from build123d import *

# Parameters (mm, degrees)
RESSALTO_EXTRUS_O1_DEPTH   = 10
ESBO_O3_W                  = 8
ESBO_O3_H                  = 6
CORTE_EXTRUS_O2_DEPTH      = 1
CORTE_EXTRUS_O2_DEPTH_BACK = 57.536791537
CORTE_EXTRUS_O1_REACH      = 63.225
ESBO_O2_R                  = 1.7
ESBO_O6_W                  = 10
ESBO_O6_H                  = 10
ESBO_O6_R                  = 1.7
RESSALTO_EXTRUS_O2_DEPTH   = 5
CORTE_EXTRUS_O5_DEPTH      = 4


with BuildPart() as part:
    # Esboço1 → Ressalto-extrusão1 (new body)
    with BuildSketch(Plane.XY):
        Polygon((0, 0), (0, -26), (6, -26), (6, -6), (26, -6), (26, -26), (32, -26), (32, 35.240055442), (56.536791537, 70.282225368), (51.621879272, 73.723683986), align=None)
        Polygon((26, 0), (26, 26.671167402), (7.324647533, 0), align=None, mode=Mode.SUBTRACT)
    extrude(amount=RESSALTO_EXTRUS_O1_DEPTH)

    # Esboço3 → Corte-extrusão2 (cut, two sides)
    with BuildSketch(Plane.ZY) as corte_extrus_o2_sk:
        with Locations((4, -16)):
            Rectangle(ESBO_O3_W, ESBO_O3_H)
    extrude(amount=CORTE_EXTRUS_O2_DEPTH, mode=Mode.SUBTRACT)
    extrude(corte_extrus_o2_sk.sketch, amount=-CORTE_EXTRUS_O2_DEPTH_BACK, mode=Mode.SUBTRACT)

    # Esboço2 → Corte-extrusão1 (cut, up to next)
    with BuildSketch(Plane(origin=(0, 0, 0), x_dir=(0, 0, 1), z_dir=(-0.819152044, 0.573576436, 0)), mode=Mode.PRIVATE) as corte_extrus_o1_sk1:
        with Locations((5, 85)):
            Circle(ESBO_O2_R)
    corte_extrus_o1_tool1 = extrude(corte_extrus_o1_sk1.sketch, amount=-CORTE_EXTRUS_O1_REACH, mode=Mode.PRIVATE) & part.part
    add(corte_extrus_o1_tool1.solids().sort_by_distance((48.753997, 69.627924, 5))[0], mode=Mode.SUBTRACT)
    # Esboço2 → Corte-extrusão1 (cut, up to next)
    with BuildSketch(Plane(origin=(0, 0, 0), x_dir=(0, 0, 1), z_dir=(-0.819152044, 0.573576436, 0)), mode=Mode.PRIVATE) as corte_extrus_o1_sk2:
        with Locations((5, 20)):
            Circle(ESBO_O2_R)
    corte_extrus_o1_tool2 = extrude(corte_extrus_o1_sk2.sketch, amount=-CORTE_EXTRUS_O1_REACH, mode=Mode.PRIVATE) & part.part
    add(corte_extrus_o1_tool2.solids().sort_by_distance((11.471529, 16.383041, 5))[0], mode=Mode.SUBTRACT)

    # Esboço6 → Ressalto-extrusão2 (add)
    with BuildSketch(Plane(origin=(0, 0, 0), x_dir=(0, 0, 1), z_dir=(-0.819152044, 0.573576436, 0))):
        with Locations((5, 85)):
            Rectangle(ESBO_O6_W, ESBO_O6_H)
        with Locations((5, 85)):
            Circle(ESBO_O6_R, mode=Mode.SUBTRACT)
        with Locations((5, 20)):
            Rectangle(ESBO_O6_W, ESBO_O6_H)
        with Locations((5, 20)):
            Circle(ESBO_O6_R, mode=Mode.SUBTRACT)
    extrude(amount=RESSALTO_EXTRUS_O2_DEPTH)

    # Esboço7 → Corte-extrusão5 (cut)
    with BuildSketch(Plane(origin=(4.914912266, -3.441458618, 0), x_dir=(0, 0, -1), z_dir=(0.819152044, -0.573576436, 0))):
        Polygon((-2.15, 83.354551733), (-2.15, 86.645448267), (-5, 88.290896534), (-7.85, 86.645448267), (-7.85, 83.354551733), (-5, 81.709103466), align=None)
        Polygon((-2.15, 18.354551733), (-2.15, 21.645448267), (-5, 23.290896534), (-7.85, 21.645448267), (-7.85, 18.354551733), (-5, 16.709103466), align=None)
    extrude(amount=-CORTE_EXTRUS_O5_DEPTH, mode=Mode.SUBTRACT)


solid = part.part
Design review of the part built by this model. Coordinates are the model's own, in mm. A direction names the side the tool comes from. Give positions to 0.01 mm unless a question says otherwise; leave off trailing zeros. Loops run counter-clockwise (first coordinate to the right, second up) from the corner with the lowest first, then second, coordinate; pieces in that order, holes last. Notation, with made-up numbers: (-16.5, -10.75) - (28.5, -10.75) arc R8 ccw to (28.5, -6.75) - close; hole circle Ø4 at (63, 53). An arc over 180 degrees is marked (long way). Write item = value, one per line.
1) Take a section at A-A on y = -8. State the section outline as (x, z) points.
Result sheet:
outline = (0, 0) - (6, 0) - (6, 10) - (0, 10) - close; (26, 0) - (32, 0) - (32, 10) - (26, 10) - close
2) Take a section at B-B on x = 20. State the section outline as (y, z) points, and give its area (3 significant figures).
Result sheet:
outline = (-6, 0) - (0, 0) - (0, 10) - (-6, 10) - close; (18.1, 0) - (28.56, 0) - (28.56, 10) - (18.1, 10) - close
area = 165 mm2
3) Take a section at C-C on x = 29. State the section outline as (y, z) points, and give its area (3 significant figures).
Result sheet:
outline = (-26, 0) - (-19, 0) - (-19, 8) - (-13, 8) - (-13, 0) - (41.42, 0) - (41.42, 10) - (-26, 10) - close
area = 626 mm2
4) Take a section at D-D on y = 59. State the section outline as (x, z) points, and give its area (3 significant figures).
Result sheet:
outline = (41.31, 0) - (48.64, 0) - (48.64, 10) - (41.31, 10) - close
area = 73.2 mm2
5) To check wall thickness, follow line 1 (Y direction, x = 14.5, z = 2.25); line 2 (X direction, y = -14, z = 8.25); line 3 (Z direction, x = 12, y = 17). State the ranges of each line that lie inside material, in increasing order.
Result sheet:
line_1 = -6 to 0, 10.25 to 12.18, 16.34 to 20.71
line_2 = 0 to 6, 26 to 32
line_3 = 0 to 3.5, 6.5 to 10
6) Draft analysis for pull direction X (two halves, no side actions). For faces 1 (the face through (3, -22, 0)), 2 (the face through (13, 12, 6)), 3 (the face through (0, -12.8, 4.9)), state which applies: +X half, -X half, draft (parallel to the pull), parting line (faces both ways), or undercut.
Result sheet:
face_1 = draft
face_2 = undercut
face_3 = -X half
7) Clearance check with flat-ended pins moving along their axes: pin 1 Ø2 at (x, z) = (25, 4.5) entering from +Y; pin 2 Ø4 at (y, z) = (7, 8) entering from -X; pin 3 Ø2 at (y, z) = (22.5, 4.5) entering from -X. State where each tip first meets the part, or that it passes through.
Result sheet:
pin_1 = 37.13
pin_2 = 3.5
pin_3 = 8.95
8) Tool access review of faces 4 (the face through (6.584, 13.701, 4.93)), 5 (the face through (16.18, 16.09, 3.56)), 6 (the face through (12.32, 21.893, 4.93)), 7 (the face through (3, -13, 4)): name each direction out of +Z, -Z, +X, -X, +Y, -Y from which nothing blocks a thin tool from reaching the whole face with its end or side.
Result sheet:
face_4 = +Z, -Z, -X
face_5 = none
face_6 = +Z, -Z, +Y
face_7 = -Z, +X, -X
